Source: CAD feature listing. Evaluate the final solid. Frame: model axes, mm. Give positions to 0.01 mm unless a question says otherwise; leave off trailing zeros. Loops run counter-clockwise (first coordinate to the right, second up) from the corner with the lowest first, then second, coordinate; pieces in that order, holes last. Notation, with made-up numbers: M -27.75,50 L 13.25,50 A26 ccw 13.25,76 Z; hole C 38.25,54.5 d10. An arc over 180 degrees is marked long. Put each result on its own line as item: value.
from build123d import *

# Parameters (mm, degrees)
BOSS_EXTRUDE1_DEPTH = 5


with BuildPart() as part:
    # Sketch2 → Boss-Extrude1 (new body)
    with BuildSketch(Plane(origin=(0, 0, 0), x_dir=(1, 0, 0), z_dir=(0, 1, 0))):
        with BuildLine():
            ThreePointArc((31.252747625, -9.809451481), (32.378051974, -4.96198779), (32.756061614, 0))
            ThreePointArc((32.756061614, 0), (32.378051974, 4.96198779), (31.252747625, 9.809451481))
            ThreePointArc((31.252747625, 9.809451481), (27.583404246, 11.425420135), (29.035359438, 15.162700114))
            ThreePointArc((29.035359438, 15.162700114), (23.162033292, 23.162033292), (15.162700114, 29.035359438))
            ThreePointArc((15.162700114, 29.035359438), (11.425420135, 27.583404246), (9.809451481, 31.252747625))
            ThreePointArc((9.809451481, 31.252747625), (0, 32.756061614), (-9.809451481, 31.252747625))
            ThreePointArc((-9.809451481, 31.252747625), (-11.425420135, 27.583404246), (-15.162700114, 29.035359438))
            ThreePointArc((-15.162700114, 29.035359438), (-23.162033292, 23.162033292), (-29.035359438, 15.162700114))
            ThreePointArc((-29.035359438, 15.162700114), (-27.583404246, 11.425420135), (-31.252747625, 9.809451481))
            ThreePointArc((-31.252747625, 9.809451481), (-32.756061614, 0), (-31.252747625, -9.809451481))
            ThreePointArc((-31.252747625, -9.809451481), (-27.583404246, -11.425420135), (-29.035359438, -15.162700114))
            ThreePointArc((-29.035359438, -15.162700114), (-23.162033292, -23.162033292), (-15.162700114, -29.035359438))
            ThreePointArc((-15.162700114, -29.035359438), (-11.425420135, -27.583404246), (-9.809451481, -31.252747625))
            ThreePointArc((-9.809451481, -31.252747625), (0, -32.756061614), (9.809451481, -31.252747625))
            ThreePointArc((9.809451481, -31.252747625), (11.425420135, -27.583404246), (15.162700114, -29.035359438))
            ThreePointArc((15.162700114, -29.035359438), (23.162033292, -23.162033292), (29.035359438, -15.162700114))
            ThreePointArc((29.035359438, -15.162700114), (27.583404246, -11.425420135), (31.252747625, -9.809451481))
        make_face()
        with BuildLine():
            Line((9.855951445, 31.372436845), (12.587804051, 37.967712456))
            ThreePointArc((12.587804051, 37.967712456), (11.630092201, 38.271934304), (10.665040579, 38.552002665))
            ThreePointArc((10.665040579, 38.552002665), (0, 36.306495263), (-10.665040579, 38.552002665))
            ThreePointArc((-10.665040579, 38.552002665), (-11.630092201, 38.271934304), (-12.587804051, 37.967712456))
            Line((-12.587804051, 37.967712456), (-9.855951445, 31.372436845))
            ThreePointArc((-9.855951445, 31.372436845), (-9.83203894, 31.312849629), (-9.809451481, 31.252747625))
            ThreePointArc((-9.809451481, 31.252747625), (0, 32.756061614), (9.809451481, 31.252747625))
            ThreePointArc((9.809451481, 31.252747625), (9.83203894, 31.312849629), (9.855951445, 31.372436845))
        make_face()
        with BuildLine():
            ThreePointArc((-17.946305339, 35.748148549), (-18.838627214, 35.286061337), (-19.719059997, 34.801705027))
            ThreePointArc((-19.719059997, 34.801705027), (-25.672569001, 25.672569001), (-34.801705027, 19.719059997))
            ThreePointArc((-34.801705027, 19.719059997), (-35.286061337, 18.838627214), (-35.748148549, 17.946305339))
            Line((-35.748148549, 17.946305339), (-29.152872937, 15.214452733))
            ThreePointArc((-29.152872937, 15.214452733), (-29.093829718, 15.189226904), (-29.035359438, 15.162700114))
            ThreePointArc((-29.035359438, 15.162700114), (-23.162033292, 23.162033292), (-15.162700114, 29.035359438))
            ThreePointArc((-15.162700114, 29.035359438), (-15.189226904, 29.093829718), (-15.214452733, 29.152872937))
            Line((-15.214452733, 29.152872937), (-17.946305339, 35.748148549))
        make_face()
        with BuildLine():
            ThreePointArc((-37.967712456, 12.587804051), (-38.271934304, 11.630092201), (-38.552002665, 10.665040579))
            ThreePointArc((-38.552002665, 10.665040579), (-36.873959465, 5.449435614), (-36.306495263, 0))
            ThreePointArc((-36.306495263, 0), (-36.873959465, -5.449435614), (-38.552002665, -10.665040579))
            ThreePointArc((-38.552002665, -10.665040579), (-38.271934304, -11.630092201), (-37.967712456, -12.587804051))
            Line((-37.967712456, -12.587804051), (-31.372436845, -9.855951445))
            ThreePointArc((-31.372436845, -9.855951445), (-31.312849629, -9.83203894), (-31.252747625, -9.809451481))
            ThreePointArc((-31.252747625, -9.809451481), (-32.756061614, 0), (-31.252747625, 9.809451481))
            ThreePointArc((-31.252747625, 9.809451481), (-31.312849629, 9.83203894), (-31.372436845, 9.855951445))
            Line((-31.372436845, 9.855951445), (-37.967712456, 12.587804051))
        make_face()
        with BuildLine():
            ThreePointArc((-15.214452733, -29.152872937), (-15.189226904, -29.093829718), (-15.162700114, -29.035359438))
            ThreePointArc((-15.162700114, -29.035359438), (-23.162033292, -23.162033292), (-29.035359438, -15.162700114))
            ThreePointArc((-29.035359438, -15.162700114), (-29.093829718, -15.189226904), (-29.152872937, -15.214452733))
            Line((-29.152872937, -15.214452733), (-35.748148549, -17.946305339))
            ThreePointArc((-35.748148549, -17.946305339), (-35.286061337, -18.838627214), (-34.801705027, -19.719059997))
            ThreePointArc((-34.801705027, -19.719059997), (-25.672569001, -25.672569001), (-19.719059997, -34.801705027))
            ThreePointArc((-19.719059997, -34.801705027), (-18.838627214, -35.286061337), (-17.946305339, -35.748148549))
            Line((-17.946305339, -35.748148549), (-15.214452733, -29.152872937))
        make_face()
        with BuildLine():
            ThreePointArc((9.855951445, -31.372436845), (9.83203894, -31.312849629), (9.809451481, -31.252747625))
            ThreePointArc((9.809451481, -31.252747625), (0, -32.756061614), (-9.809451481, -31.252747625))
            ThreePointArc((-9.809451481, -31.252747625), (-9.83203894, -31.312849629), (-9.855951445, -31.372436845))
            Line((-9.855951445, -31.372436845), (-12.587804051, -37.967712456))
            ThreePointArc((-12.587804051, -37.967712456), (-11.630092201, -38.271934304), (-10.665040579, -38.552002665))
            ThreePointArc((-10.665040579, -38.552002665), (0, -36.306495263), (10.665040579, -38.552002665))
            ThreePointArc((10.665040579, -38.552002665), (11.630092201, -38.271934304), (12.587804051, -37.967712456))
            Line((12.587804051, -37.967712456), (9.855951445, -31.372436845))
        make_face()
        with BuildLine():
            ThreePointArc((29.152872937, -15.214452733), (29.093829718, -15.189226904), (29.035359438, -15.162700114))
            ThreePointArc((29.035359438, -15.162700114), (23.162033292, -23.162033292), (15.162700114, -29.035359438))
            ThreePointArc((15.162700114, -29.035359438), (15.189226904, -29.093829718), (15.214452733, -29.152872937))
            Line((15.214452733, -29.152872937), (17.946305339, -35.748148549))
            ThreePointArc((17.946305339, -35.748148549), (18.838627214, -35.286061337), (19.719059997, -34.801705027))
            ThreePointArc((19.719059997, -34.801705027), (25.672569001, -25.672569001), (34.801705027, -19.719059997))
            ThreePointArc((34.801705027, -19.719059997), (35.286061337, -18.838627214), (35.748148549, -17.946305339))
            Line((35.748148549, -17.946305339), (29.152872937, -15.214452733))
        make_face()
        with BuildLine():
            ThreePointArc((34.987322012, -11.353285907), (33.319161403, -5.785231712), (32.756061614, 0))
            ThreePointArc((32.756061614, 0), (32.378051974, -4.96198779), (31.252747625, -9.809451481))
            ThreePointArc((31.252747625, -9.809451481), (31.312849629, -9.83203894), (31.372436845, -9.855951445))
            Line((31.372436845, -9.855951445), (34.987322012, -11.353285907))
        make_face()
        with BuildLine():
            ThreePointArc((38.552002665, 10.665040579), (38.271934304, 11.630092201), (37.967712456, 12.587804051))
            Line((37.967712456, 12.587804051), (34.987322012, 11.353285907))
            ThreePointArc((34.987322012, 11.353285907), (33.319161403, 5.785231712), (32.756061614, 0))
            ThreePointArc((32.756061614, 0), (33.319161403, -5.785231712), (34.987322012, -11.353285907))
            Line((34.987322012, -11.353285907), (37.967712456, -12.587804051))
            ThreePointArc((37.967712456, -12.587804051), (38.271934304, -11.630092201), (38.552002665, -10.665040579))
            ThreePointArc((38.552002665, -10.665040579), (36.306495263, 0), (38.552002665, 10.665040579))
        make_face()
        with BuildLine():
            ThreePointArc((32.756061614, 0), (33.319161403, 5.785231712), (34.987322012, 11.353285907))
            Line((34.987322012, 11.353285907), (31.372436845, 9.855951445))
            ThreePointArc((31.372436845, 9.855951445), (31.312849629, 9.83203894), (31.252747625, 9.809451481))
            ThreePointArc((31.252747625, 9.809451481), (32.378051974, 4.96198779), (32.756061614, 0))
        make_face()
        with BuildLine():
            Line((29.152872937, 15.214452733), (35.748148549, 17.946305339))
            ThreePointArc((35.748148549, 17.946305339), (35.286061337, 18.838627214), (34.801705027, 19.719059997))
            ThreePointArc((34.801705027, 19.719059997), (25.672569001, 25.672569001), (19.719059997, 34.801705027))
            ThreePointArc((19.719059997, 34.801705027), (18.838627214, 35.286061337), (17.946305339, 35.748148549))
            Line((17.946305339, 35.748148549), (15.214452733, 29.152872937))
            ThreePointArc((15.214452733, 29.152872937), (15.189226904, 29.093829718), (15.162700114, 29.035359438))
            ThreePointArc((15.162700114, 29.035359438), (23.162033292, 23.162033292), (29.035359438, 15.162700114))
            ThreePointArc((29.035359438, 15.162700114), (29.093829718, 15.189226904), (29.152872937, 15.214452733))
        make_face()
    extrude(amount=BOSS_EXTRUDE1_DEPTH)


solid = part.part
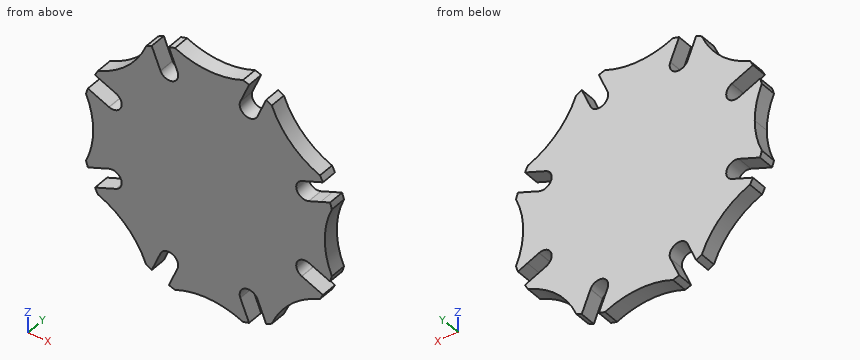
1. Material intervals for line 1 (X direction, y = 2.75, z = 32); line 2 (X direction, y = 0.95, z = 30), sorted ascending. Write a range as from..to.
Found:
line 1: -21..-16.39, -10.12..10.12, 16.39..21
line 2: -22.17..-15.57, -9.65..9.65, 15.57..22.17
2. Section query A-A (x = -33.5). Output: boundary loops of the cut face in (y, z).
Found:
outline: M 0,-20.26 L 5,-20.26 L 5,-17.02 L 0,-17.02 Z; M 0,-10.74 L 5,-10.74 L 5,10.74 L 0,10.74 Z; M 0,17.02 L 5,17.02 L 5,20.26 L 0,20.26 Z
3. Section query C-C (x = -23). Output: boundary loops of the cut face in (y, z), plus the area to 3 significant figures.
Found:
outline: M 0,-28.8 L 5,-28.8 L 5,28.8 L 0,28.8 Z
area: 288 mm^2
4. Contact query for flat-ended pins moving along their axis: P1, Ø1, axis at y = 2, z = -11.5, coming from the -X side; P2, Ø6, axis at x = -6, z = -27.5, coming from the -Y side; P3, Ø1, axis at x = 24, y = 2.5, coming from the +Z side; P4, Ø1.5, axis at y = 4.5, z = 5, coming from the -X side. Output: stop coordinate, or through.
Found:
P1: x = -38.46
P2: y = 0
P3: z = 28.13
P4: x = -36.94
5. Section query B-B (z = 4). Output: boundary loops of the cut face in (x, y).
Found:
outline: M -36.61,0 L 36.61,0 L 36.61,5 L -36.61,5 Z
